from build123d import *

# Parameters (mm, degrees)
SKETCH3_R           = 1.5
BOSS_EXTRUDE3_DEPTH = 80
CUT_EXTRUDE1_DEPTH  = 180.357185527
SKETCH5_W           = 3.1
SKETCH5_H           = 12
CUT_EXTRUDE2_DEPTH  = 180.357185527
FILLET1_R           = 4


with BuildPart() as part:
    # Sketch3 → Boss-Extrude3 (new body)
    with BuildSketch(Plane(origin=(0, 0, 0), x_dir=(0, 0, -1), z_dir=(1, 0, 0))):
        Polygon((0, 160), (13, 160), (13, 151), (3, 151), (3, 9), (12, 9), (12, 0), (0, 0), align=None)
        with Locations((8, 155)):
            Circle(SKETCH3_R, mode=Mode.SUBTRACT)
        with Locations((8, 5)):
            Circle(SKETCH3_R, mode=Mode.SUBTRACT)
    extrude(amount=BOSS_EXTRUDE3_DEPTH)

    # Sketch4 → Cut-Extrude1 (cut, through all)
    with BuildSketch(Plane.XY):
        Polygon((11.5, 117), (11.5, 129), (68.5, 129), (68.5, 117), (72, 117), (72, 67), (68.5, 67), (68.5, 20), (11.5, 20), (11.5, 67), (8, 67), (8, 117), align=None)
    extrude(amount=-CUT_EXTRUDE1_DEPTH, mode=Mode.SUBTRACT)

    # Sketch5 → Cut-Extrude2 (cut, through all)
    with BuildSketch(Plane(origin=(0, 0, 0), x_dir=(1, 0, 0), z_dir=(0, 1, 0))):
        with Locations((78.45, 9)):
            Rectangle(SKETCH5_W, SKETCH5_H)
        with Locations((1.55, 9)):
            Rectangle(SKETCH5_W, SKETCH5_H)
    extrude(amount=CUT_EXTRUDE2_DEPTH, mode=Mode.SUBTRACT)

    # Fillet1
    fillet1_edges = [part.edges().sort_by_distance(p)[0] for p in [
        (40, 151, -13),
        (40, 9, -12),
    ]]
    fillet(fillet1_edges, radius=FILLET1_R)


solid = part.part
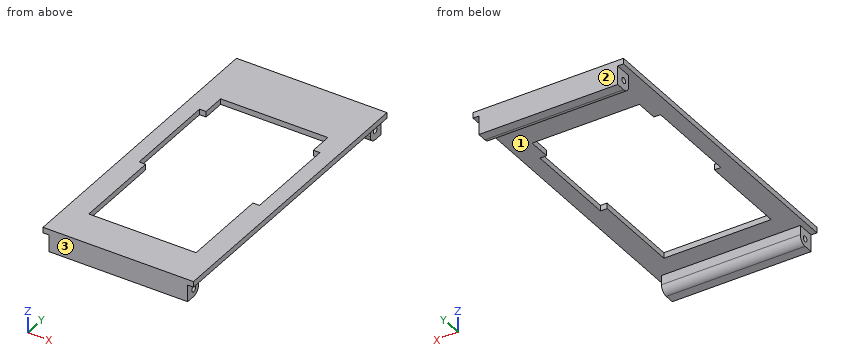
The listing builds one solid part. Answer for the finished solid, in the listing's coordinates (mm). Face numbers are marked on the shaded views. Coordinates: 2 decimals unless noted, no trailing zeros. Loops run counter-clockwise (first coordinate to the right, second up) from the corner with the lowest first, then second, coordinate; pieces in that order, holes last. Notation, with made-up numbers: M 74,59 L 100,59 A14 ccw 100,86 Z; hole C 48,53 d11. An arc over 180 degrees is marked long. Answer in a Markdown table with one row per item.
1) Find the intervals of material crossed by probe 1 along Y at (x, z) = (18, -8); probe 2 along Z at (x, y) = (32, 155); probe 3 along Y at (x, z) = (44.5, -6.25), in increasing order.
Answers below:
| item | result |
|---|---|
| probe 1 | 0 to 3.5, 6.5 to 9, 151 to 153.5, 156.5 to 160 |
| probe 2 | -13 to -9.5, -6.5 to 0 |
| probe 3 | 0 to 9, 151 to 160 |
2) Given pin 1 (5 mm diameter, centred on y = 5, z = -8, fed in from -X); pin 2 (1.5 mm diameter, centred on x = 13, y = 137, fed in from -Z), each flat-ended and moving along its own axis, determine where each tip first touches the part or whether it passes through.
Answers below:
| item | result |
|---|---|
| pin 1 | x = 3.1 |
| pin 2 | z = -3 |
3) Find section C-C (y = 71.5). Determine the outline of the cut face in (x, z), then the cut area to 3 significant figures.
Answers below:
| item | result |
|---|---|
| outline | M 0,-3 L 8,-3 L 8,0 L 0,0 Z; M 72,-3 L 80,-3 L 80,0 L 72,0 Z |
| area | 48.0 mm^2 |
4) Determine the mould class of the marked faces 1, 2 and 3 for opening direction Y: released by +Y, released by -Y, zero draft, split by the parting line, or undercut.
Answers below:
| item | result |
|---|---|
| face 1 | undercut |
| face 2 | released by +Y |
| face 3 | released by -Y |
5) Find section B-B (z = -4.75). Determine the outline of the cut face in (x, y).
Answers below:
| item | result |
|---|---|
| outline | M 3.1,0 L 76.9,0 L 76.9,9 L 3.1,9 Z; M 3.1,151 L 76.9,151 L 76.9,160 L 3.1,160 Z |
6) Find section D-D (y = 146). Determine the outline of the cut face in (x, z).
Answers below:
| item | result |
|---|---|
| outline | M 0,-3 L 80,-3 L 80,0 L 0,0 Z |
7) Find section A-A (x = 61). Determine the outline of the cut face in (y, z), then the cut area to 3 significant figures.
Answers below:
| item | result |
|---|---|
| outline | M 0,-12 L 5,-12 A4 ccw 9,-8 L 9,-3 L 20,-3 L 20,0 L 0,0 Z; M 129,-3 L 151,-3 L 151,-9 A4 ccw 155,-13 L 160,-13 L 160,0 L 129,0 Z; hole C 5,-8 d3; hole C 155,-8 d3 |
| area | 303 mm^2 |
